from build123d import *

# Parameters (mm, degrees)
ESQUISSE1_W                  = 12.75
ESQUISSE1_H                  = 5.77
BASE_EXTRUSION_DEPTH         = 3
ESQUISSE2_W                  = 1.5
ESQUISSE2_H                  = 0.4
ESQUISSE2_W_2                = 3.4
ENL_V_MAT_EXTRU_1_DEPTH      = 3.885
ENL_V_MAT_EXTRU_1_DEPTH_BACK = 3.885
COQUE1_T                     = -0.8
ESQUISSE3_W                  = 0.9
ESQUISSE3_H                  = 0.44
BOSS_EXTRU_1_DEPTH           = 3.75
ESQUISSE4_W                  = 11.75
ESQUISSE4_H                  = 4.77
ESQUISSE4_W_2                = 11.15
ESQUISSE4_H_2                = 4.17
BOSS_EXTRU_2_DEPTH           = 0.8
ENL_V_MAT_EXTRU_2_DEPTH      = 0.5
SYM_TRIE2_COPY_1_DEPTH       = 0.5
CHANFREIN1_SIZE              = 0.1
ESQUISSE6_W                  = 1.9
ESQUISSE6_H                  = 0.45
BOSS_EXTRU_3_DEPTH           = 0.5
CHANFREIN2_SIZE              = 0.4
CHANFREIN2_OF_SYM_TRIE3_SIZE = 0.4
ESQUISSE7_R                  = 1
ENL_V_MAT_EXTRU_3_DEPTH      = 3.885
ENL_V_MAT_EXTRU_3_DEPTH_BACK = 3.885


with BuildPart() as part:
    # Esquisse1 → Base-Extrusion (new body)
    with BuildSketch(Plane.XY):
        Rectangle(ESQUISSE1_W, ESQUISSE1_H)
    extrude(amount=-BASE_EXTRUSION_DEPTH)

    # Esquisse2 → Enlèv. mat.-Extru.1 (cut, two sides)
    with BuildSketch(Plane(origin=(0, 0, 0), x_dir=(1, 0, 0), z_dir=(0, 1, 0))) as enl_v_mat_extru_1_sk:
        with Locations((-5.065, 2.8)):
            Rectangle(ESQUISSE2_W, ESQUISSE2_H)
        with Locations((5.065, 2.8)):
            Rectangle(ESQUISSE2_W, ESQUISSE2_H)
        with Locations((0, 2.8)):
            Rectangle(ESQUISSE2_W_2, ESQUISSE2_H)
    extrude(amount=ENL_V_MAT_EXTRU_1_DEPTH, mode=Mode.SUBTRACT)
    extrude(enl_v_mat_extru_1_sk.sketch, amount=-ENL_V_MAT_EXTRU_1_DEPTH_BACK, mode=Mode.SUBTRACT)

    # Coque1
    coque1_openings = [part.faces().sort_by_distance(p)[0] for p in [
        (0, 0, 0),
    ]]
    offset(amount=COQUE1_T, openings=coque1_openings, kind=Kind.INTERSECTION)

    # Esquisse3 → Boss.-Extru.1 (add)
    with BuildSketch(Plane(origin=(0, 0, -2.6), x_dir=(-1, 0, 0), z_dir=(0, 0, -1))):
        with Locations((-5.065, 0)):
            Rectangle(ESQUISSE3_W, ESQUISSE3_H)
        with Locations((5.065, 0)):
            Rectangle(ESQUISSE3_W, ESQUISSE3_H)
        Rectangle(ESQUISSE3_W, ESQUISSE3_H)
    extrude(amount=BOSS_EXTRU_1_DEPTH)

    # Esquisse4 → Boss.-Extru.2 (add)
    with BuildSketch(Plane.XY):
        Rectangle(ESQUISSE4_W, ESQUISSE4_H)
        Rectangle(ESQUISSE4_W_2, ESQUISSE4_H_2, mode=Mode.SUBTRACT)
    extrude(amount=BOSS_EXTRU_2_DEPTH)

    # Esquisse5 → Enlèv. mat.-Extru.2 (cut)
    with BuildSketch(Plane(origin=(0, 2.885, 0), x_dir=(1, 0, 0), z_dir=(0, 1, 0))):
        with BuildLine():
            Line((3, 0), (0, 0))
            Line((0, 0), (0, 2))
            Line((0, 2), (1.75, 2))
            Line((1.75, 2), (1.75, 1.25))
            ThreePointArc((1.75, 1.25), (2.116116524, 0.366116524), (3, 0))
        make_face()
    enl_v_mat_extru_2 = extrude(amount=-ENL_V_MAT_EXTRU_2_DEPTH, mode=Mode.SUBTRACT)

    # Symétrie1: Enlèv. mat.-Extru.2 across plane
    add(enl_v_mat_extru_2.mirror(Plane(origin=(0, 0, 0), x_dir=(0, 0, 1), z_dir=(1, 0, 0))), mode=Mode.SUBTRACT)

    # Symétrie2: Enlèv. mat.-Extru.2 across plane
    add(enl_v_mat_extru_2.mirror(Plane.ZX), mode=Mode.SUBTRACT)

    # Symétrie2 copy 1 sketch → Symétrie2 copy 1 (cut)
    with BuildSketch(Plane(origin=(0, -2.885, 0), x_dir=(-1, 0, 0), z_dir=(0, -1, 0))):
        with BuildLine():
            Line((3, 0), (0, 0))
            Line((0, 0), (0, 2))
            Line((0, 2), (1.75, 2))
            Line((1.75, 2), (1.75, 1.25))
            ThreePointArc((1.75, 1.25), (2.116116524, 0.366116524), (3, 0))
        make_face()
    extrude(amount=-SYM_TRIE2_COPY_1_DEPTH, mode=Mode.SUBTRACT)

    # Chanfrein1
    chanfrein1_edges = [part.edges().sort_by_distance(p)[0] for p in [
        (5.875, -2.385, 0.4),
        (5.875, 2.385, 0.4),
        (-5.875, 2.385, 0.4),
        (-5.875, -2.385, 0.4),
    ]]
    chamfer(chanfrein1_edges, length=CHANFREIN1_SIZE)

    # Esquisse6 → Boss.-Extru.3 (add)
    with BuildSketch(Plane(origin=(0, 2.385, 0), x_dir=(-1, 0, 0), z_dir=(0, 1, 0))):
        with Locations((0, -1.025)):
            Rectangle(ESQUISSE6_W, ESQUISSE6_H)
    boss_extru_3 = extrude(amount=BOSS_EXTRU_3_DEPTH)

    # Chanfrein2
    chanfrein2_edges = [part.edges().sort_by_distance(p)[0] for p in [
        (0, 2.885, -0.8),
    ]]
    chamfer(chanfrein2_edges, length=CHANFREIN2_SIZE)

    # Symétrie3: Boss.-Extru.3 across plane
    add(boss_extru_3.mirror(Plane.ZX))

    # Chanfrein2 of Symétrie3
    chanfrein2_of_sym_trie3_edges = [part.edges().sort_by_distance(p)[0] for p in [
        (0, -2.885, -0.8),
    ]]
    chamfer(chanfrein2_of_sym_trie3_edges, length=CHANFREIN2_OF_SYM_TRIE3_SIZE)

    # Esquisse7 → Enlèv. mat.-Extru.3 (cut, two sides)
    with BuildSketch(Plane(origin=(0, 0, 0), x_dir=(1, 0, 0), z_dir=(0, 1, 0))) as enl_v_mat_extru_3_sk:
        with Locations((3.25, 1.5)):
            Circle(ESQUISSE7_R)
        with Locations((-3.25, 1.5)):
            Circle(ESQUISSE7_R)
    extrude(amount=ENL_V_MAT_EXTRU_3_DEPTH, mode=Mode.SUBTRACT)
    extrude(enl_v_mat_extru_3_sk.sketch, amount=-ENL_V_MAT_EXTRU_3_DEPTH_BACK, mode=Mode.SUBTRACT)


solid = part.part
Geometry check sheet. Reference: the model listing, model coordinates, mm. A direction names the side the tool comes from. Give positions to 0.01 mm unless a question says otherwise; leave off trailing zeros. Order: outer loops, then holes, each group sorted by start corner. A loop starts at its lowest first (then second) coordinate and runs counter-clockwise, first axis right, second up. Notation, with made-up numbers: M 52.25,-4.75 L 68.25,-4.75 A7 ccw 68.25,2.25 Z; hole C 22.5,25.25 d3. An arc over 180 degrees is marked long. Use a Markdown table: item, result.
Item 1: Section check B-B (z = -1.5). State how many separate pieces and enclosed holes the cut face has, and give its area (3 significant figures).
Answers follow:
| item | result |
|---|---|
| separate pieces | 4 |
| enclosed holes | 0 |
| area | 17.2 mm2 |
Item 2: Section check A-A (x = -3.25). Record the cut outline in (y, z) (3 decimals), and give its area (4 significant figures).
Answers follow:
| item | result |
|---|---|
| outline | M -2.885,-3 L 2.885,-3 L 2.885,-2.5 L -2.885,-2.5 Z; M -2.885,-0.5 L -2.085,-0.5 L -2.085,0.8 L -2.385,0.8 L -2.385,0 L -2.885,0 Z; M 2.085,-0.5 L 2.885,-0.5 L 2.885,0 L 2.385,0 L 2.385,0.8 L 2.085,0.8 Z |
| area | 4.165 mm2 |
Item 3: Material ranges on line 1 along Y through (x, z) = (5, -0.25) (3 decimals); line 2 along X through (y, z) = (-0.35, -1.5) (3 decimals); line 3 along Z through (x, y) = (-3.25, 2.3), recorded low to high.
Answers follow:
| item | result |
|---|---|
| line 1 | y = -2.885 to -2.085, 2.085 to 2.885 |
| line 2 | x = -6.375 to -5.575, 5.575 to 6.375 |
| line 3 | z = -3 to -2.5, -0.5 to 0.8 |
Item 4: Depth check by flat-ended pin: P1, Ø2, axis at x = -2.5, y = -0.5, coming from the +Z side; P2, Ø1.5, axis at x = 0, z = -4.5, coming from the -Y side. Enter the tip coordinate at first touch or a pass-through.
Answers follow:
| item | result |
|---|---|
| P1 | stops at z = -1.8 |
| P2 | stops at y = -0.22 |
Item 5: Draft check along Y on faces 1 (the cylindrical face through (-2.106, 2.638, -0.376)), 2 (the flat face through (0, -0.22, -4)), 3 (the flat face through (0, 0, -1.8)). Enter one of: +Y half, -Y half, draft (parallel to the pull), parting line (faces both ways), or undercut.
Answers follow:
| item | result |
|---|---|
| face 1 | draft |
| face 2 | -Y half |
| face 3 | undercut |
Item 6: Tool access check on faces 4 (the cylindrical face through (-2.106, -2.638, -0.376)), 5 (the flat face through (-5, 0, -1.8)), 6 (the cylindrical face through (2.106, 2.638, -0.376)), 7 (the flat face through (6.1, 0.2, 0)). Record the directions out of +Z, -Z, +X, -X, +Y, -Y that give a thin tool (end or side, any length) a straight path to the whole face; none if there is none.
Answers follow:
| item | result |
|---|---|
| face 4 | +Z, -Y |
| face 5 | +Z |
| face 6 | +Z, +Y |
| face 7 | +Z, +X |
Item 7: Section check D-D (z = -0.25). Record the cut outline in (x, y) (3 decimals), and give its area (3 significant figures).
Answers follow:
| item | result |
|---|---|
| outline | M -6.375,-2.885 L -2.25,-2.885 L -2.25,-2.385 L 2.25,-2.385 L 2.25,-2.885 L 6.375,-2.885 L 6.375,2.885 L 2.25,2.885 L 2.25,2.385 L -2.25,2.385 L -2.25,2.885 L -6.375,2.885 Z; hole M -5.575,-2.085 L 5.575,-2.085 L 5.575,2.085 L -5.575,2.085 Z |
| area | 22.6 mm2 |
